Check sheet for the modelled part. Datum: model origin and axes. Units: mm. A direction names the side the tool comes from. Round coordinates to 2 decimals unless told otherwise and drop trailing zeros. Loops run counter-clockwise (first coordinate to the right, second up) from the corner with the lowest first, then second, coordinate; pieces in that order, holes last. Notation, with made-up numbers: (32.25, -29.5) - (68.25, -29.5) arc R29 cw to (68.25, -3.5) - close; hole circle Ø10 at (51.25, 44.5). An arc over 180 degrees is marked (long way). Put each result on its own line as item: value. Start each with the question number.
```python
from build123d import *

# Parameters (mm, degrees)
SKETCH1_W           = 40
SKETCH1_H           = 125
BOSS_EXTRUDE1_DEPTH = 6
SKETCH2_W           = 5.5
SKETCH2_H           = 15
SKETCH2_W_2         = 12
SKETCH2_H_2         = 89
CUT_EXTRUDE1_DEPTH  = 132.381124976
SKETCH3_W           = 6
SKETCH3_H           = 37
CUT_EXTRUDE2_DEPTH  = 132.381124976


with BuildPart() as part:
    # Sketch1 → Boss-Extrude1 (new body)
    with BuildSketch(Plane.XY):
        with Locations((20, 62.5)):
            Rectangle(SKETCH1_W, SKETCH1_H)
    extrude(amount=BOSS_EXTRUDE1_DEPTH)

    # Sketch2 → Cut-Extrude1 (cut, through all)
    with BuildSketch(Plane.XY.offset(6)):
        with Locations((8.75, 117.5)):
            Rectangle(SKETCH2_W, SKETCH2_H)
        with Locations((6, 44.5)):
            Rectangle(SKETCH2_W_2, SKETCH2_H_2)
    extrude(amount=-CUT_EXTRUDE1_DEPTH, mode=Mode.SUBTRACT)

    # Sketch3 → Cut-Extrude2 (cut, through all)
    with BuildSketch(Plane.XY.offset(6)):
        with Locations((15, 47.5)):
            Rectangle(SKETCH3_W, SKETCH3_H)
    extrude(amount=-CUT_EXTRUDE2_DEPTH, mode=Mode.SUBTRACT)


solid = part.part
```
Q1. Cross-section at D-D on x = 10. Enter the section's corners in (y, z), and give its area (3 significant figures).
Q2. Cross-section at C-C on y = 40.5. Enter the section's corners in (x, z), and give its area (3 significant figures).
Q3. Material ranges on line 1 (X direction, y = 113.5, z = 3); line 2 (Y direction, x = 13.5, z = 5); line 3 (X direction, y = 74, z = 3.05), recorded low to high. Write a range as from..to.
Q4. Cross-section at A-A on y = 116.5. Enter the section's corners in (x, z), and give its area (3 significant figures).
Q5. Depth check by flat-ended pin: pin 1 Ø1.8 at (y, z) = (49, 3) entering from -X; pin 2 Ø1.8 at (x, z) = (3.5, 4) entering from -Y; pin 3 Ø1.5 at (x, y) = (20, 67.5) entering from -Z; pin 4 Ø3 at (y, z) = (9.5, 3.5) entering from -X. Enter the tip coordinate at first touch or a pass-through.
Q6. Cross-section at B-B on z = 4.65. Enter the section's corners in (x, y).
Q7. Set-up check for faces 1 (the face through (18, 47, 3)), 2 (the face through (6, 117, 3)), 3 (the face through (12, 14, 3)): record each of +Z, -Z, +X, -X, +Y, -Y from which the full face is reachable in a straight line by a thin tool's end or side.
Q8. Draft check along X on faces 4 (the face through (9, 110, 3)), 5 (the face through (24, 63, 6)), 6 (the face through (12, 77, 3)), 7 (the face through (11.5, 117, 3)). Enter one of: +X half, -X half, draft (parallel to the pull), parting line (faces both ways), or undercut.
Answer list:
1. outline: (89, 0) - (110, 0) - (110, 6) - (89, 6) - close
1. area: 126 mm2
2. outline: (18, 0) - (40, 0) - (40, 6) - (18, 6) - close
2. area: 132 mm2
3. line 1: x = 0..6, 11.5..40
3. line 2: y = 0..29, 66..125
3. line 3: x = 12..40
4. outline: (0, 0) - (6, 0) - (6, 6) - (0, 6) - close; (11.5, 0) - (40, 0) - (40, 6) - (11.5, 6) - close
4. area: 207 mm2
5. pin 1: stops at x = 18
5. pin 2: stops at y = 89
5. pin 3: stops at z = 0
5. pin 4: stops at x = 12
6. outline: (0, 89) - (12, 89) - (12, 66) - (18, 66) - (18, 29) - (12, 29) - (12, 0) - (40, 0) - (40, 125) - (11.5, 125) - (11.5, 110) - (6, 110) - (6, 125) - (0, 125) - close
7. face 1: +Z, -Z, -X
7. face 2: +Z, -Z, +Y
7. face 3: +Z, -Z, -X, -Y
8. face 4: undercut
8. face 5: draft
8. face 6: -X half
8. face 7: undercut
